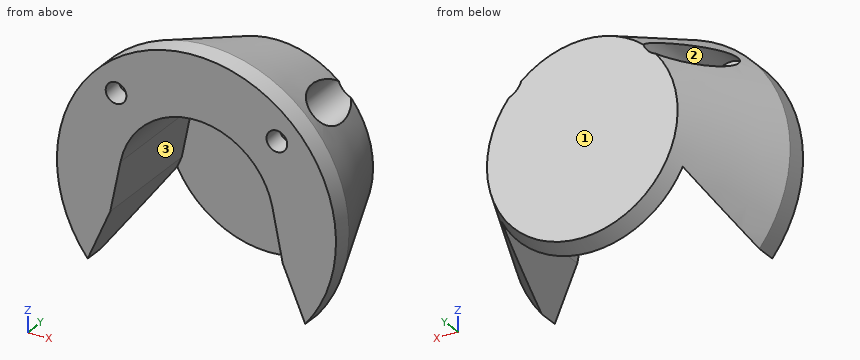
```python
from build123d import *

# Parameters (mm, degrees)
SKETCH5_R          = 2
CUT_EXTRUDE2_DEPTH = 46.639894829
SKETCH6_R          = 4
CUT_EXTRUDE3_DEPTH = 22
SKETCH7_R          = 4.5
CUT_EXTRUDE4_DEPTH = 22
CUT_EXTRUDE5_DEPTH = 22


with BuildPart() as part:
    # Sketch2 → Revolve1 (revolve)
    with BuildSketch(Plane(origin=(0, 0, 0), x_dir=(0, 0, -1), z_dir=(1, 0, 0)), mode=Mode.PRIVATE) as revolve1_sk:
        Polygon((-18.45, 25), (-27, 4), (-27, 0), (-15, 0), (-15, 22), (0, 22), (0, 25), align=None)
    revolve(revolve1_sk.sketch.rotate(Axis((0, 0, 0), (0, 1, 0)), 180), axis=Axis((0, 0, 0), (0, 1, 0)))

    # Sketch5 → Cut-Extrude2 (cut, through all)
    with BuildSketch(Plane(origin=(0, 25, 0), x_dir=(1, 0, 0), z_dir=(0, 1, 0))):
        with Locations(Location((-15.556349186, -15.556349186, 0), (0, 0, 270))):
            Circle(SKETCH5_R)
        with Locations(Location((15.556349186, -15.556349186, 0), (0, 0, 270))):
            Circle(SKETCH5_R)
    extrude(amount=-CUT_EXTRUDE2_DEPTH, mode=Mode.SUBTRACT)

    # Sketch6 → Cut-Extrude3 (cut)
    with BuildSketch(Plane(origin=(0, 4, 0), x_dir=(-1, 0, 0), z_dir=(0, -1, 0))):
        with Locations(Location((15.556349186, -15.556349186, 0), (0, 0, 90))):
            Circle(SKETCH6_R)
        with Locations(Location((-15.556349186, -15.556349186, 0), (0, 0, 90))):
            Circle(SKETCH6_R)
    extrude(amount=-CUT_EXTRUDE3_DEPTH, mode=Mode.SUBTRACT)

    # Sketch7 → Cut-Extrude4 (cut)
    with BuildSketch(Plane(origin=(0, 0, 0), x_dir=(-1, 0, 0), z_dir=(0, -1, 0))):
        with Locations(Location((15.556349186, 15.556349186, 0), (0, 0, 90))):
            Circle(SKETCH7_R)
        with Locations(Location((-15.556349186, 15.556349186, 0), (0, 0, 90))):
            Circle(SKETCH7_R)
    extrude(amount=-CUT_EXTRUDE4_DEPTH, mode=Mode.SUBTRACT)

    # Sketch10 → Cut-Extrude5 (cut)
    with BuildSketch(Plane.XZ):
        with BuildLine():
            Line((-14.704067619, 2.964860106), (-16.680641023, -6.837851641))
            Line((-16.680641023, -6.837851641), (-21.048400418, -16.910494961))
            ThreePointArc((-21.048400418, -16.910494961), (-18.731046773, -19.446024961), (-16.110526631, -21.666816371))
            ThreePointArc((-16.110526631, -21.666816371), (0, -27), (16.110526631, -21.666816371))
            ThreePointArc((16.110526631, -21.666816371), (18.731046773, -19.446024961), (21.048400418, -16.910494961))
            Line((21.048400418, -16.910494961), (16.680641023, -6.837851641))
            Line((16.680641023, -6.837851641), (14.704067619, 2.964860106))
            ThreePointArc((14.704067619, 2.964860106), (0, 15), (-14.704067619, 2.964860106))
        make_face()
    extrude(amount=-CUT_EXTRUDE5_DEPTH, mode=Mode.SUBTRACT)


solid = part.part
```
The listing builds one solid part. Answer for the finished solid, in the listing's coordinates (mm). Face numbers are marked on the shaded views. A direction names the side the tool comes from. Give positions to 0.01 mm unless a question says otherwise; leave off trailing zeros. Order: outer loops, then holes, each group sorted by start corner. A loop starts at its lowest first (then second) coordinate and runs counter-clockwise, first axis right, second up. Notation, with made-up numbers: (5.5, 44.5) - (62.5, 44.5) arc R17 ccw to (62.5, 67.5) - close; hole circle Ø1 at (0, -6). An arc over 180 degrees is marked (long way). Use one line per item in the form item = value. Start each with the question number.
(1) A cutting plane is placed at D-D, the plane z = 0. Write down the section's boundary in (x, y), then the cut area to 3 significant figures.
(2) Flat-ended cylindrical pins translate along their axes: pin 1 Ø8 at (x, y) = (7, 19.5) entering from +Z; pin 2 Ø3 at (x, z) = (15.56, 15.56) entering from -Y; pin 3 Ø1 at (y, z) = (7, 17.5) entering from -X; pin 4 Ø4 at (x, z) = (-14.5, 14.5) entering from +Y. Find the tip coordinate at first contact, or state that the pin passes through.
(3) A cutting plane is placed at B-B, the plane x = 0. Write down the section's boundary in (y, z).
(4) A cutting plane is placed at A-A, the plane y = 10. Write down the section's boundary in (x, z), then the cut area to 3 significant figures.
(5) Consider line 1 (X direction, y = 9.5, z = 12); line 2 (X direction, y = 2, z = 17); line 3 (Y direction, x = -11, z = -8). Determine where each line is inside the solid, lowest interval first. Write a range as from..to.
(6) A cutting plane is placed at C-C, the plane y = 2.25. Write down the section's boundary in (x, z), then the cut area to 3 significant figures.
(7) For the marked faces 1, 2 and 3, determine the directions among +Z, -Z, +X, -X, +Y, -Y from which every point of the face is accessible in a straight line to the end or side of a thin tool.
Ans:
q1.outline = (-27, 0) - (-15.3, 0) - (-15.3, 22) - (15.3, 22) - (15.3, 0) - (27, 0) - (27, 4) - (18.45, 25) - (-18.45, 25) - (-27, 4) - close
q1.area = 497 mm^2
q2.pin_1 = 21.53
q2.pin_2 = through
q2.pin_3 = -19.46
q2.pin_4 = 4
q3.outline = (0, 15) - (22, 15) - (22, -19.67) - (25, -18.45) - (25, 18.45) - (4, 27) - (0, 27) - close
q4.outline = (-19.93, -14.34) - (-16.68, -6.84) - (-14.7, 2.96) arc R15 cw to (14.7, 2.96) - (16.68, -6.84) - (19.93, -14.34) arc R24.56 ccw to (19.51, 14.92) arc R4 cw (long way) to (14.92, 19.51) arc R24.56 ccw to (-14.92, 19.51) arc R4 cw (long way) to (-19.51, 14.92) arc R24.56 ccw to start
q4.area = 674 mm^2
q5.line_1 = -21.66..-17.39, -13.73..-9, 9..13.73, 17.39..21.66
q5.line_2 = -20.98..-16.94, -14.17..14.17, 16.94..20.98
q5.line_3 = 22..25
q6.outline = (-21.05, -16.91) - (-16.68, -6.84) - (-14.7, 2.96) arc R15 cw to (14.7, 2.96) - (16.68, -6.84) - (21.05, -16.91) arc R27 ccw (long way) to start; hole circle Ø4 at (-15.56, 15.56); hole circle Ø4 at (15.56, 15.56)
q6.area = 1,020 mm^2
q7.face_1 = +Z, -Z, +X, -X, +Y
q7.face_2 = +Y
q7.face_3 = -Z, -Y
